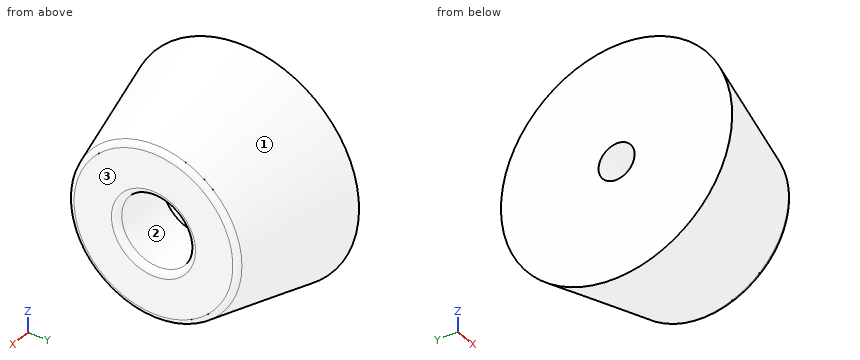
Autodesk Inventor part; units mm, degrees
ref_plane "YZ Plane" through (0, 0, 0) normal (1, 0, 0) x (0, 1, 0)
ref_plane "XZ Plane" through (0, 0, 0) normal (0, 1, 0) x (-1, 0, 0)
ref_plane "XY Plane" through (0, 0, 0) normal (0, 0, 1) x (1, 0, 0)
sketch "Sketch2" plane through (0, 0, 0) normal (0, 1, 0) x (-1, 0, 0)
  line L0 (0, 0) -> (0, -14)
  line L1 (0, -14) -> (21, -19.25)
  line L2 (21, -19.25) -> (21, 0)
  line L3 (21, 0) -> (0, 0)
  dimension "d1" = 14
  dimension "d2" = 21
  dimension "d3" = 19.25
revolve "Revolution1" add sketch "Sketch2" angle 360 about axis through (-21, 0, 0) along (1, 0, 0)
sketch "Sketch3" plane through (-21, 0, 0) normal (-1, 0, 0) x (0, 0, 1)
  circle A0 centre (0, 0) radius 3
  dimension "d5" = 6
extrude "Extrusion1" cut sketch "Sketch3" against normal through all
sketch "Sketch4" plane through (0, 0, 0) normal (1, 0, 0) x (0, 0, -1)
  circle A0 centre (0, 0) radius 6
  dimension "d8" = 12
extrude "Extrusion2" cut sketch "Sketch4" against normal blind 10.5
fillet "Fillet1" radius 1 2 edges at (0, 0, 14) (0, 0, 6)
properties part number "Rubberfoot"
Verification items for the finished model (mm, model axes). Face numbers are marked on the shaded views. Coordinates: 2 decimals unless noted, no trailing zeros. Write each loop counter-clockwise with the first axis right and the second up, starting at its lowest first coordinate (ties: lowest second). Pieces come first, ordered by that corner, then holes. Notation, with made-up numbers: (-29, -13.75) -> (25, -13.75) arc R12 cw to (25, -1.75) -> close; hole circle Ø4 at (82, 83). An arc over 180 degrees is marked (long way). One line per item, written item: value. Start each with the question number.
Q1. Mould release check, pull along Z, two halves, no side actions. Record for the marked faces 1, 2 and 3: pulls with the +Z half, pulls with the -Z half, needs draft (parallel to the pull), parting line crosses it, or undercut.
Q2. Cross-section at D-D on x = -14.75. Enter the section's corners in (y, z) (1 decimal), and give its area (3 significant figures).
Q3. Thickness scan on L1, parallel to Z at x = -19, y = 1.5; L2, parallel to X at y = 3, z = 5; L3, parallel to Z at x = -15.5, y = -2.5. Record the ranges inside material, lowest first. Write a range as from..to.
Q4. Cross-section at C-C on x = -8.5. Enter the section's corners in (y, z) (3 decimals), and give its area (3 significant figures).
Q5. Cross-section at A-A on y = 0. Enter the section's corners in (x, z), and give its area (3 significant figures).
Q6. Go/stop test with flat-tipped pins: P1, Ø10, axis at x = -4, z = 4.5, coming from the -Y side; P2, Ø3.5, axis at y = 1.5, z = 3, coming from the +X side; P3, Ø4, axis at x = -10, y = 5.5, coming from the +Z side. Record where each tip stops, or that it passes through.
Checked values:
1. face 1: parting line crosses it
1. face 2: undercut
1. face 3: needs draft
2. outline: circle Ø35.4 at (0, 0); hole circle Ø6 at (0, 0)
2. area: 955 mm²
3. L1: z = -18.69..-2.6, 2.6..18.69
3. L2: x = -21..-10.5
3. L3: z = -17.7..-1.66, 1.66..17.7
4. outline: circle Ø32.25 at (0, 0); hole circle Ø12 at (0, 0)
4. area: 704 mm²
5. outline: (-21, -19.25) -> (-0.76, -14.19) arc R1 ccw to (0, -13.22) -> (0, -7) arc R1 ccw to (-1, -6) -> (-10.5, -6) -> (-10.5, -3) -> (-21, -3) -> close; (-21, 3) -> (-10.5, 3) -> (-10.5, 6) -> (-1, 6) arc R1 ccw to (0, 7) -> (0, 13.22) arc R1 ccw to (-0.76, 14.19) -> (-21, 19.25) -> close
5. area: 509 mm²
6. P1: stops at y = -15.96
6. P2: stops at x = -10.5
6. P3: stops at z = 16.35
